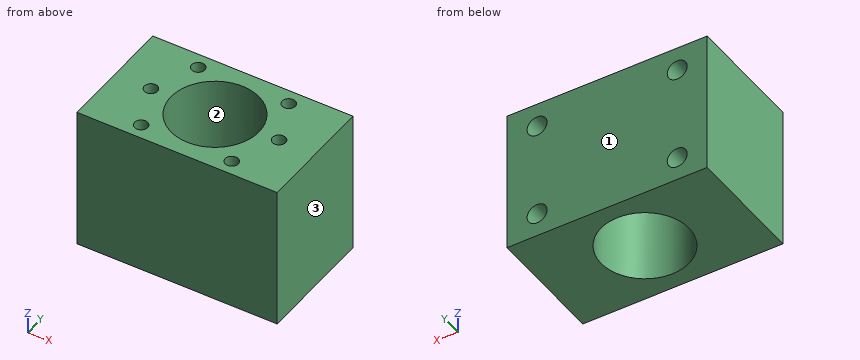
```python
from build123d import *

# Parameters (mm, degrees)
SKETCH2_W                   = 50
SKETCH2_H                   = 30
SKETCH2_R                   = 11
BOSS_EXTRUDE1_DEPTH         = 36
TAP_DRILL_FOR_M4_TAP1_D     = 3.3
TAP_DRILL_FOR_M4_TAP1_DEPTH = 7.008579979
TAP_DRILL_FOR_M4_TAP1_TIP   = 0.991420021
SKETCH5_R                   = 2.5
CUT_EXTRUDE1_DEPTH          = 12


with BuildPart() as part:
    # Sketch2 → Boss-Extrude1 (new body)
    with BuildSketch(Plane.XY):
        Rectangle(SKETCH2_W, SKETCH2_H)
        Circle(SKETCH2_R, mode=Mode.SUBTRACT)
    extrude(amount=BOSS_EXTRUDE1_DEPTH)

    # Tap Drill for M4 Tap1
    with Locations(Plane.XY.offset(36)):
        with Locations((11.313708499, 11.313708499), (-16, 0), (-11.313708499, 11.313708499), (-11.313708499, -11.313708499), (11.313708499, -11.313708499), (16, 0)):
            Hole(TAP_DRILL_FOR_M4_TAP1_D / 2, depth=TAP_DRILL_FOR_M4_TAP1_DEPTH)
            with Locations((0, 0, -(TAP_DRILL_FOR_M4_TAP1_DEPTH + TAP_DRILL_FOR_M4_TAP1_TIP / 2))):  # 118° drill point
                Cone(0, TAP_DRILL_FOR_M4_TAP1_D / 2, TAP_DRILL_FOR_M4_TAP1_TIP, mode=Mode.SUBTRACT)

    # Sketch5 → Cut-Extrude1 (cut)
    with BuildSketch(Plane(origin=(0, 15, 0), x_dir=(1, 0, 0), z_dir=(0, 1, 0))):
        with Locations(Location((-17.5, -6, 0), (0, 0, 270))):
            Circle(SKETCH5_R)
        with Locations(Location((17.5, -6, 0), (0, 0, 270))):
            Circle(SKETCH5_R)
        with Locations(Location((17.5, -30, 0), (0, 0, 270))):
            Circle(SKETCH5_R)
        with Locations(Location((-17.5, -30, 0), (0, 0, 270))):
            Circle(SKETCH5_R)
    extrude(amount=-CUT_EXTRUDE1_DEPTH, mode=Mode.SUBTRACT)


solid = part.part
```
Check sheet for the modelled part. Datum: model origin and axes. Units: mm. Face numbers are marked on the shaded views. Give positions to 0.01 mm unless a question says otherwise; leave off trailing zeros. Order: outer loops, then holes, each group sorted by start corner. A loop starts at its lowest first (then second) coordinate and runs counter-clockwise, first axis right, second up. Notation, with made-up numbers: (47.5, -33) -> (86.5, -33) arc R30 cw to (86.5, -9) -> close; hole circle Ø6 at (69.25, 34.25). An arc over 180 degrees is marked (long way). Return JSON: item names as keys, results as strings.
1. Cross-section at C-C, the plane y = -3.25. Record the cut outline in (x, z), plus the area to 3 significant figures.
From the geometry:
{"outline": "(-25, 0) -> (-10.51, 0) -> (-10.51, 36) -> (-25, 36) -> close; (10.51, 0) -> (25, 0) -> (25, 36) -> (10.51, 36) -> close", "area": "1,040 mm^2"}
2. Cross-section at B-B, the plane z = 6. Record the cut outline in (x, y), plus the area to 4 significant figures.
From the geometry:
{"outline": "(-25, -15) -> (25, -15) -> (25, 15) -> (20, 15) -> (20, 3) -> (15, 3) -> (15, 15) -> (-15, 15) -> (-15, 3) -> (-20, 3) -> (-20, 15) -> (-25, 15) -> close; hole circle Ø22 at (0, 0)", "area": "1,000 mm^2"}
3. Mould release check, pull along Y, two halves, no side actions. Record for the marked faces 1, 2 and 3: +Y half, -Y half, draft (parallel to the pull), parting line (faces both ways), or undercut.
From the geometry:
{"face 1": "+Y half", "face 2": "undercut", "face 3": "draft"}
4. Material ranges on probe 1 along Y at (x, z) = (0, 22); probe 2 along X at (y, z) = (6, 6); probe 3 along X at (y, z) = (6.25, 30), recorded low to high. Write a range as [from, to].
From the geometry:
{"probe 1": "[-15, -11], [11, 15]", "probe 2": "[-25, -20], [-15, -9.22], [9.22, 15], [20, 25]", "probe 3": "[-25, -20], [-15, -9.05], [9.05, 15], [20, 25]"}
5. Cross-section at D-D, the plane z = 31.5. Record the cut outline in (x, y), plus the area to 3 significant figures.
From the geometry:
{"outline": "(-25, -15) -> (25, -15) -> (25, 15) -> (19.5, 15) -> (19.5, 3) -> (15.5, 3) -> (15.5, 15) -> (-15.5, 15) -> (-15.5, 3) -> (-19.5, 3) -> (-19.5, 15) -> (-25, 15) -> close; hole circle Ø3.3 at (-16, 0); hole circle Ø3.3 at (-11.31, -11.31); hole circle Ø3.3 at (-11.31, 11.31); hole circle Ø22 at (0, 0); hole circle Ø3.3 at (11.31, -11.31); hole circle Ø3.3 at (11.31, 11.31); hole circle Ø3.3 at (16, 0)", "area": "973 mm^2"}
6. Cross-section at A-A, the plane y = 6.5. Record the cut outline in (x, z).
From the geometry:
{"outline": "(-25, 0) -> (-8.87, 0) -> (-8.87, 36) -> (-25, 36) -> close; (8.87, 0) -> (25, 0) -> (25, 36) -> (8.87, 36) -> close; hole circle Ø5 at (-17.5, 6); hole circle Ø5 at (-17.5, 30); hole circle Ø5 at (17.5, 6); hole circle Ø5 at (17.5, 30)"}
7. Go/stop test with flat-tipped pins: P1, Ø2, axis at x = 19.5, y = 11.5, coming from the -Z side; P2, Ø4, axis at x = 17.5, z = 30, coming from the +Y side; P3, Ø3, axis at x = -11.31, y = 11.31, coming from the +Z side; P4, Ø2.5, axis at x = -16, y = 0, coming from the +Z side. Record where each tip stops, or that it passes through.
From the geometry:
{"P1": "z = 0", "P2": "y = 3", "P3": "z = 28.9", "P4": "z = 28.75"}
